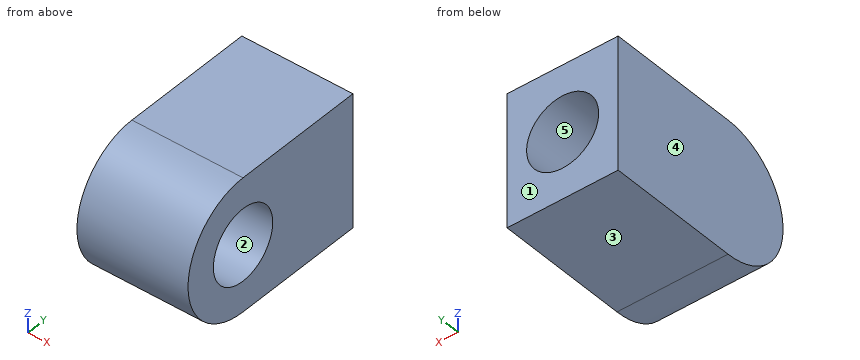
Autodesk Inventor part; units mm, degrees
ref_plane "YZ Plane" through (0, 0, 0) normal (1, 0, 0) x (0, 1, 0)
ref_plane "XZ Plane" through (0, 0, 0) normal (0, 1, 0) x (-1, 0, 0)
ref_plane "XY Plane" through (0, 0, 0) normal (0, 0, 1) x (1, 0, 0)
sketch "Esboço1" plane through (0, 0, 0) normal (1, 0, 0) x (0, 1, 0)
  line L0 (0, 0) -> (5.9987, 0)
  line L1 (5.9987, 0) -> (5.9987, -6)
  line L2 (5.9987, -6) -> (-0.0013, -6)
  arc A0 (0, 0) -> (-0.0013, -6) centre (-0.0007, -3) ccw
  dimension "d0" = 6
  dimension "d1" = 6
  dimension "d3" = 3
extrude "Extrusão1" add sketch "Esboço1" along normal blind 5
sketch "Esboço2" plane through (5, 0, 0) normal (1, 0, 0) x (0, 0, -1)
  arc A0 (0, 0) -> (6, -0.0013) centre (3, -0.0007) ccw
hole "Furo1" at (5, -0.0007, -3) direction (-1, 0, 0) diameter 3.242 depth 4
sketch "Esboço3" plane through (0, 5.9987, 0) normal (0, 1, 0) x (1, 0, 0)
  line L0 (5, 0) -> (5, 6)
  line L1 (0, 6) -> (0, 0)
  point P0 (2.5, 3)
hole "Furo2" at (2.5, 5.9987, -3) direction (0, -1, 0) diameter 3.242 depth 4
properties part number "CONECTOR U-L"
Part model, mm, in its own coordinate system. Face numbers are marked on the shaded views. A direction names the side the tool comes from. Coordinates: 2 decimals unless noted, no trailing zeros. Loops run counter-clockwise (first coordinate to the right, second up) from the corner with the lowest first, then second, coordinate; pieces in that order, holes last. Notation, with made-up numbers: (-6, 21.5) - (-2, 21.5) arc R23 ccw to (-2, 44.5) - close; hole circle Ø10 at (60, 49.25). An arc over 180 degrees is marked (long way). Write each question's results on one line, items separated by ' | '. Start each with the question number.
Q1. Slice it at C-C on x = 2.8. Give the cut face in (y, z).
Q2. Which spindle directions (+Z, -Z, +X, -X, +Y, -Y) get a long thin tool onto all of the face, cutting with end or side? Do the marked faces 1 and 2. Say none if no direction does.
Q3. Slice it at A-A on z = -3. Give the cut face in (x, y), and give its area (3 significant figures).
Q4. Slice it at D-D on x = 3.95. Give the cut face in (y, z).
Q5. Probe line 1 along Y through (x, z) = (2.6, -3); line 2 along X through (y, z) = (3.5, -3); line 3 along Z through (x, y) = (2.5, 5.1). List the from-to ranges inside material, lowest first.
Q6. Slice it at B-B on y = 2.25. Give the cut face in (x, z).
Q7. Two-plate mould, pull along Z, no slides. Class the marked faces 3, 4 and 5: +Z half, -Z half, draft (parallel to the pull), parting line (faces both ways), or undercut.
Answer:
1) outline: (0, -6) - (6, -6) - (6, -4.59) - (2, -4.59) - (2, -1.41) - (6, -1.41) - (6, 0) - (0, 0) arc R3 ccw to start; hole circle Ø3.24 at (0, -3)
2) face 1: +Z, -Z, +X, -X, +Y | face 2: +X
3) outline: (0, -3) - (5, -3) - (5, -1.62) - (1, -1.62) - (1, 1.62) - (5, 1.62) - (5, 6) - (4.12, 6) - (4.12, 2) - (0.88, 2) - (0.88, 6) - (0, 6) - close | area: 19.1 mm2
4) outline: (0, -6) - (6, -6) - (6, -3.72) - (2, -3.72) - (2, -2.28) - (6, -2.28) - (6, 0) - (0, 0) arc R3 ccw to start; hole circle Ø3.24 at (0, -3)
5) line 1: y = -3 to -1.62, 1.62 to 2 | line 2: x = 0 to 0.88, 4.12 to 5 | line 3: z = -6 to -4.62, -1.38 to 0
6) outline: (0, -6) - (5, -6) - (5, 0) - (0, 0) - close; hole circle Ø3.24 at (2.5, -3)
7) face 3: -Z half | face 4: draft | face 5: undercut
